```python
from build123d import *

# Parameters (mm, degrees)
F0_W         = 781.2
F0_H         = 998.2
F1_DEPTH     = 20
F2_R         = 50.8
F4_DEPTH     = 25.4
F5_T1_DEPTH  = 20
F5_T3_DEPTH  = 401
F6_W         = 260.4
F6_H         = 46.8
F7_DEPTH     = 25.4
F8_W         = 150
F8_H         = 40
F9_DEPTH     = 20.0010001
F10_T1_DEPTH = 20


# Not quite as in the source:
# - a fillet or chamfer that OpenCascade refuses, or shapes differently, is made with other operations: its cross-section is extruded or revolved along the edge and cut away or added


with BuildPart() as f1:
    # F0 (on Front) → F1 (new body)
    with BuildSketch(Plane.XZ):
        Rectangle(F0_W, F0_H)
    extrude(amount=F1_DEPTH)

    # F2
    f2_edges = [f1.edges().sort_by_distance(p)[0] for p in [
        (-390.6, -10, 499.1),
        (390.6, -10, 499.1),
        (390.6, -10, -499.1),
        (-390.6, -10, -499.1),
    ]]
    fillet(f2_edges, radius=F2_R)

    # F3 (on Front) → F4 (cut)
    with BuildSketch(Plane.XZ):
        Polygon((303.8, 412.3), (-303.8, 412.3), (-303.8, -151.9), (-130.2, -151.9), (-130.2, -412.3), (130.2, -412.3), (130.2, -151.9), (303.8, -151.9), align=None)
    extrude(amount=F4_DEPTH, mode=Mode.SUBTRACT)

    # F5: fillet of radius 76.2 on 6 edges, made by hand

    # F5_s2 → F5_t1 (join)
    with BuildSketch(Plane.XZ):
        with BuildLine():
            add(Edge.make_bspline(
                [(-303.8, -75.7), (-303.8, -151.9), (-227.6, -151.9)],
                knots=[0, 0, 0, 1, 1, 1], degree=2, weights=[1, 1, 1]))
            Line((-227.6, -151.9), (-303.8, -151.9))
            Line((-303.8, -151.9), (-303.8, -75.7))
        make_face()
        with BuildLine():
            add(Edge.make_bspline(
                [(-130.2, -336.1), (-130.2, -412.3), (-54, -412.3)],
                knots=[0, 0, 0, 1, 1, 1], degree=2, weights=[1, 1, 1]))
            Line((-54, -412.3), (-130.2, -412.3))
            Line((-130.2, -412.3), (-130.2, -336.1))
        make_face()
        with BuildLine():
            add(Edge.make_bspline(
                [(227.6, -151.9), (303.8, -151.9), (303.8, -75.7)],
                knots=[0, 0, 0, 1, 1, 1], degree=2, weights=[1, 1, 1]))
            Line((303.8, -75.7), (303.8, -151.9))
            Line((303.8, -151.9), (227.6, -151.9))
        make_face()
        with BuildLine():
            add(Edge.make_bspline(
                [(54, -412.3), (130.2, -412.3), (130.2, -336.1)],
                knots=[0, 0, 0, 1, 1, 1], degree=2, weights=[1, 1, 1]))
            Line((130.2, -336.1), (130.2, -412.3))
            Line((130.2, -412.3), (54, -412.3))
        make_face()
    extrude(amount=F5_T1_DEPTH)

    # F5_s4 → F5_t3 (cut)
    with BuildSketch(Plane.XZ.offset(-190.5)):
        with BuildLine():
            add(Edge.make_bspline(
                [(-206.4, -151.9), (-130.2, -151.9), (-130.2, -228.1)],
                knots=[0, 0, 0, 1, 1, 1], degree=2, weights=[1, 1, 1]))
            Line((-130.2, -228.1), (-130.2, -151.9))
            Line((-130.2, -151.9), (-206.4, -151.9))
        make_face()
        with BuildLine():
            add(Edge.make_bspline(
                [(130.2, -228.1), (130.2, -151.9), (206.4, -151.9)],
                knots=[0, 0, 0, 1, 1, 1], degree=2, weights=[1, 1, 1]))
            Line((206.4, -151.9), (130.2, -151.9))
            Line((130.2, -151.9), (130.2, -228.1))
        make_face()
    extrude(amount=F5_T3_DEPTH, mode=Mode.SUBTRACT)

    # F6 (on Front) → F7 (cut)
    with BuildSketch(Plane.XZ):
        with Locations((0, 455.7)):
            Rectangle(F6_W, F6_H)
    extrude(amount=-F7_DEPTH, mode=Mode.SUBTRACT)

    # F8 (on face) → F9 (cut, through all)
    with BuildSketch(Plane.XZ.offset(20)):
        with Locations((0, 459.1)):
            Rectangle(F8_W, F8_H)
    extrude(amount=-F9_DEPTH, mode=Mode.SUBTRACT)

    # F10: fillet of radius 25.4 on 4 edges, made by hand

    # F10_s2 → F10_t1 (join)
    with BuildSketch(Plane.XZ):
        with BuildLine():
            add(Edge.make_bspline(
                [(-49.6, 479.1), (-75, 479.1), (-75, 453.7)],
                knots=[0, 0, 0, 1, 1, 1], degree=2, weights=[1, 1, 1]))
            Line((-75, 453.7), (-75, 479.1))
            Line((-75, 479.1), (-49.6, 479.1))
        make_face()
        with BuildLine():
            add(Edge.make_bspline(
                [(-75, 464.5), (-75, 439.1), (-49.6, 439.1)],
                knots=[0, 0, 0, 1, 1, 1], degree=2, weights=[1, 1, 1]))
            Line((-49.6, 439.1), (-75, 439.1))
            Line((-75, 439.1), (-75, 464.5))
        make_face()
        with BuildLine():
            add(Edge.make_bspline(
                [(49.6, 479.1), (75, 479.1), (75, 453.7)],
                knots=[0, 0, 0, 1, 1, 1], degree=2, weights=[1, 1, 1]))
            Line((75, 453.7), (75, 479.1))
            Line((75, 479.1), (49.6, 479.1))
        make_face()
        with BuildLine():
            add(Edge.make_bspline(
                [(49.6, 439.1), (75, 439.1), (75, 464.5)],
                knots=[0, 0, 0, 1, 1, 1], degree=2, weights=[1, 1, 1]))
            Line((75, 464.5), (75, 439.1))
            Line((75, 439.1), (49.6, 439.1))
        make_face()
    extrude(amount=F10_T1_DEPTH)


solid = f1.part
```
For this review, take the finished solid that the model builds, in its own axes (mm). A direction names the side the tool comes from. Give positions to 0.01 mm unless a question says otherwise; leave off trailing zeros. Write each loop counter-clockwise with the first axis right and the second up, starting at its lowest first coordinate (ties: lowest second). Pieces come first, ordered by that corner, then holes. Notation, with made-up numbers: M -19,20.5 L 36,20.5 A22 cw 36,54.5 Z; hole C -6,-39.75 d1. An arc over 180 degrees is marked long. Answer as a JSON object with one key per item and string values. Group by question number.
Item 1: For probe 1 along X at (y, z) = (-9, 206); probe 2 along Z at (x, y) = (-16, -2.5); probe 3 along Z at (x, y) = (53, -1.25), list the stretches that pass through material, from the lowest coordinate up. Write a range as [from, to].
Item 2: Tool access review of faces 1 (the cylindrical face through (375.324, -10.14, -484.614)), 2 (the flat face through (130.2, -10, -283)): name each direction out of +Z, -Z, +X, -X, +Y, -Y from which nothing blocks a thin tool from reaching the whole face with its end or side.
Item 3: Consider section C-C on y = -16. Count the separate pieces of the cut face and the enclosed holes in it, plus the area to 3 significant figures.
Item 4: Draft analysis for pull direction X (two halves, no side actions). For faces 3 (the cylindrical face through (376.114, -10.14, 483.824)), 4 (the flat face through (179, -20, -215)), 5 (the flat face through (-130.2, -10, -281)), state which applies: +X half, -X half, draft (parallel to the pull), parting line (faces both ways), or undercut.
Item 5: Consider section B-B on z = -279.5. Write out the cut boundary in (x, y).
Item 6: Consider section A-A on z = 352.5. Write out the cut boundary in (x, y).
Check result:
{
 "1": {"probe 1": "x = [-390.6, -303.8], [303.8, 390.6]", "probe 2": "z = [-499.1, -412.3], [412.3, 439.1], [479.1, 499.1]", "probe 3": "z = [-499.1, -412.3], [412.3, 439.22], [478.98, 499.1]"},
 "2": {"face 1": "-Z, +X, +Y, -Y", "face 2": "+Y, -Y"},
 "3": {"separate pieces": "1", "enclosed holes": "2", "area": "363,000 mm^2"},
 "4": {"face 3": "+X half", "face 4": "draft", "face 5": "undercut"},
 "5": {"outline": "M -390.6,-20 L -130.2,-20 L -130.2,0 L -390.6,0 Z; M 130.2,-20 L 390.6,-20 L 390.6,0 L 130.2,0 Z"},
 "6": {"outline": "M -390.6,-20 L -303.8,-20 L -303.8,0 L -390.6,0 Z; M 303.8,-20 L 390.6,-20 L 390.6,0 L 303.8,0 Z"}
}
